For this review, use the dimensioned drawing (mm, ordinates from the lowest corner) and the shaded views. Coordinates: 2 decimals unless noted, no trailing zeros. Loops run counter-clockwise (first coordinate to the right, second up) from the corner with the lowest first, then second, coordinate; pieces in that order, holes last. Notation, with made-up numbers: (72.5, -30.5) - (103.5, -30.5) arc R22 cw to (103.5, -15.5) - close; hole circle Ø10 at (27, 8). An arc over 180 degrees is marked (long way). Answer in a Markdown table with one row per item. Add a question column.
(1) We need section A-A on x = 8.5. Write out the cut boundary in (y, z) (1 decimal).
(2) We need section B-B on z = 5.25. Write out the cut boundary in (x, y).
(3) We need section D-D on x = 0.5. Write out the cut boundary in (y, z) (1 decimal), plus the area to 3 significant figures.
(4) We need section C-C on y = 6.75. Write out the cut boundary in (x, z).
(5) For P1, Ø4, axis at x = 2.5, z = 1.5, coming from the -Y side; P2, Ø2, axis at x = 2, y = 8.5, coming from the -Z side, all flat-tipped, find the tip position at first contact; note any pin that passes through.
(6) For line 1 along Z through (x, y) = (8.75, 4); line 2 along Y through (x, z) = (8.25, 1.75); line 3 along Z through (x, y) = (2.5, 8.75), list the stretches that pass through material, from the lowest coordinate up.
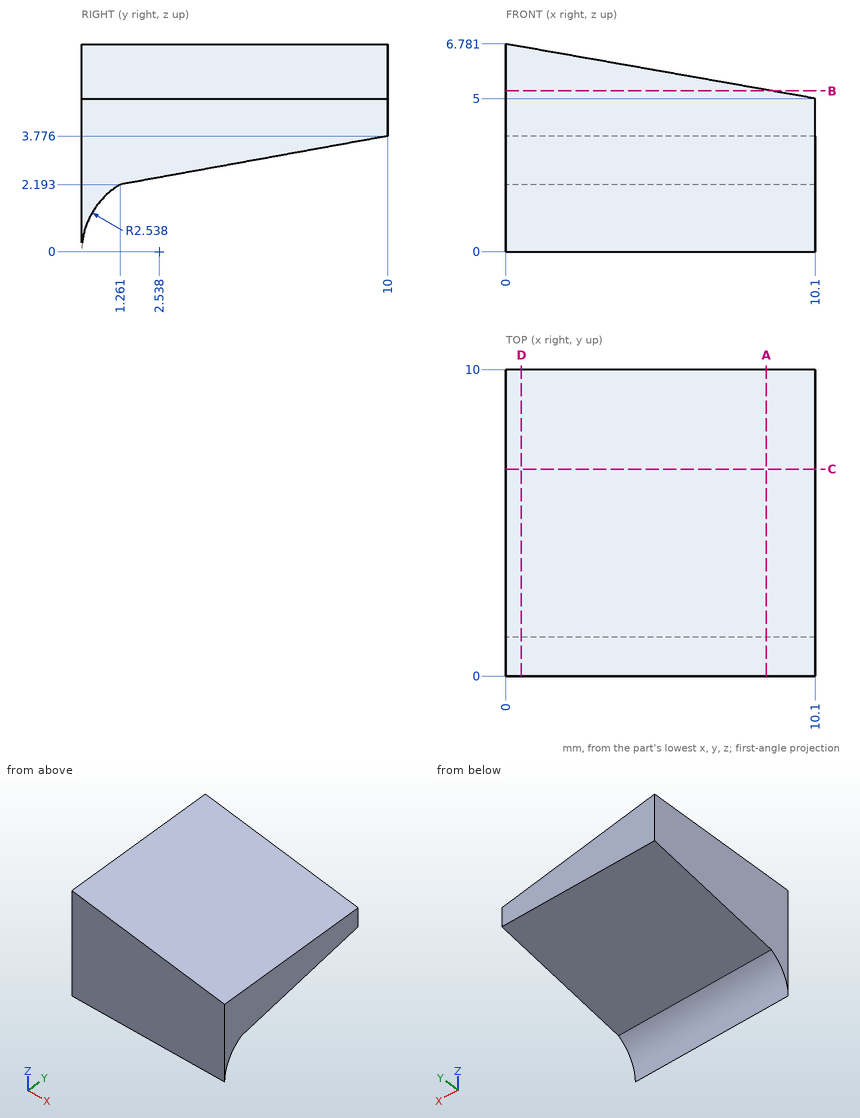
Outcome:
| question | item | result |
|---|---|---|
| 1 | outline | (0, 0) arc R2.5 cw to (1.3, 2.2) - (10, 3.8) - (10, 5.3) - (0, 5.3) - close |
| 2 | outline | (0, 0) - (8.68, 0) - (8.68, 10) - (0, 10) - close |
| 3 | outline | (0, 0) arc R2.5 cw to (1.3, 2.2) - (10, 3.8) - (10, 6.7) - (0, 6.7) - close |
| 3 | area | 38.9 mm² |
| 4 | outline | (0, 3.19) - (10.1, 3.19) - (10.1, 5) - (0, 6.78) - close |
| 5 | P1 | y = 0 |
| 5 | P2 | z = 3.32 |
| 6 | line 1 | 2.69 to 5.24 |
| 6 | line 2 | 0 to 0.7 |
| 6 | line 3 | 3.55 to 6.34 |
